Check sheet for the modelled part. Datum: model origin and axes. Units: mm. Round coordinates to 2 decimals unless told otherwise and drop trailing zeros. Loops run counter-clockwise (first coordinate to the right, second up) from the corner with the lowest first, then second, coordinate; pieces in that order, holes last. Notation, with made-up numbers: (57, -12) - (63, -12) arc R10 cw to (63, -2) - close; hole circle Ø3 at (-17.5, -16). An arc over 180 degrees is marked (long way). Return JSON: item names as keys, results as strings.
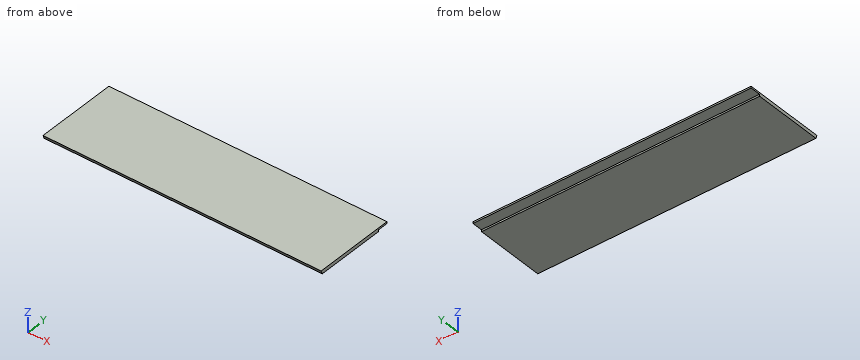
from build123d import *

# Parameters (mm, degrees)
SKETCH1_W           = 1262
SKETCH1_H           = 370.62
BOSS_EXTRUDE1_DEPTH = 16
SKETCH2_W           = 1262
SKETCH2_H           = 47.7
CUT_EXTRUDE1_DEPTH  = 8.1
CUT_EXTRUDE2_DEPTH  = 1276.633096192


with BuildPart() as part:
    # Sketch1 → Boss-Extrude1 (new body)
    with BuildSketch(Plane.XY):
        Rectangle(SKETCH1_W, SKETCH1_H)
    extrude(amount=BOSS_EXTRUDE1_DEPTH)

    # Sketch2 → Cut-Extrude1 (cut)
    with BuildSketch(Plane(origin=(0, 0, 0), x_dir=(-1, 0, 0), z_dir=(0, 0, -1))):
        with Locations((0, 161.46)):
            Rectangle(SKETCH2_W, SKETCH2_H)
    extrude(amount=-CUT_EXTRUDE1_DEPTH, mode=Mode.SUBTRACT)

    # Sketch3 → Cut-Extrude2 (cut, through all)
    with BuildSketch(Plane(origin=(631, 0, 0), x_dir=(0, 0, -1), z_dir=(1, 0, 0))):
        Polygon((-16, -185.31), (0, -179.168175439), (0, -185.31), align=None)
    extrude(amount=-CUT_EXTRUDE2_DEPTH, mode=Mode.SUBTRACT)


solid = part.part
Q1. Sectioned sample at A-A (x = 83). Enter the section's corners in (y, z), plus the area to 3 significant figures.
Answer key:
{"outline": "(-185.31, 16) - (-179.17, 0) - (137.61, 0) - (137.61, 8.1) - (185.31, 8.1) - (185.31, 16) - close", "area": "5,490 mm²"}
Q2. Depth check by flat-ended pin: P1, Ø6.5, axis at x = 60.5, z = 4, coming from the +Y side; P2, Ø4, axis at x = 95.5, z = 2, coming from the -Y side. Enter the tip coordinate at first touch or a pass-through.
Answer key:
{"P1": "stops at y = 137.61", "P2": "stops at y = -180.7"}
Q3. Sectioned sample at C-C (z = 5). Enter the section's corners in (x, y), plus the area to 3 significant figures.
Answer key:
{"outline": "(-631, -181.09) - (631, -181.09) - (631, 137.61) - (-631, 137.61) - close", "area": "402,000 mm²"}
Q4. Scan lines: probe 1 along Y at (x, z) = (396.5, 15.5); probe 2 along Y at (x, z) = (-315, 15). Record each from-to range of solid material in increasing order. Write a range as [from, to].
Answer key:
{"probe 1": "y = [-185.12, 185.31]", "probe 2": "y = [-184.93, 185.31]"}
Q5. Sectioned sample at B-B (y = 152). Enter the section's corners in (x, z), plus the area to 3 significant figures.
Answer key:
{"outline": "(-631, 8.1) - (631, 8.1) - (631, 16) - (-631, 16) - close", "area": "9,970 mm²"}
